```python
from build123d import *

# Parameters (mm, degrees)
F0_W     = 460
F0_H     = 170
F1_DEPTH = 30
F2_W     = 420
F2_H     = 130
F3_DEPTH = 30
F4_W     = 450
F4_H     = 150
F5_DEPTH = 10
F6_W     = 420
F6_H     = 0.1
F7_DEPTH = 0.1


with BuildPart() as f1:
    # F0 (on Top) → F1 (new body)
    with BuildSketch(Plane.XY):
        with Locations((41.152232, -18.289462)):
            Rectangle(F0_W, F0_H)
    extrude(amount=F1_DEPTH)

    # F2 (on face) → F3 (cut, through all)
    with BuildSketch(Plane.XY.offset(30)):
        with Locations((41.152232, -18.289462)):
            Rectangle(F2_W, F2_H)
    extrude(amount=-F3_DEPTH, mode=Mode.SUBTRACT)

    # F4 (on face) → F5 (cut)
    with BuildSketch(Plane(origin=(0, 0, 0), x_dir=(1, 0, 0), z_dir=(0, 0, -1))):
        with Locations((36.152232, 18.289462)):
            Rectangle(F4_W, F4_H)
    extrude(amount=-F5_DEPTH, mode=Mode.SUBTRACT)

    # F6 (on face) → F7 (cut)
    with BuildSketch(Plane(origin=(0, -83.289462, 0), x_dir=(-1, 0, 0), z_dir=(0, 1, 0))):
        with Locations((-41.152232, 20.05)):
            Rectangle(F6_W, F6_H)
    extrude(amount=-F7_DEPTH, mode=Mode.SUBTRACT)


solid = f1.part
```
The model under review builds one solid part; all positions refer to its coordinate system, in mm. A direction names the side the tool comes from. Round coordinates to 2 decimals unless told otherwise and drop trailing zeros. Order: outer loops, then holes, each group sorted by start corner. A loop starts at its lowest first (then second) coordinate and runs counter-clockwise, first axis right, second up. Notation, with made-up numbers: (47, 83.25) -> (78, 83.25) arc R21 ccw to (78, 112.25) -> close; hole circle Ø6 at (9, -31). An arc over 180 degrees is marked (long way). One line per item, written item: value. Start each with the question number.
Q1. Take a section at C-C (x = -43.5). Write out the cut boundary in (y, z), and give its area (4 significant figures).
Q2. Wall thickness on line 1 (Y direction, x = 46.5, z = 22.5); line 2 (X direction, y = -42, z = 26.25); line 3 (Y direction, x = -61, z = 5.5): over which ranges is each line inside the solid? List them lowest first.
Q3. Take a section at B-B (z = 15.25). Write out the cut boundary in (x, y).
Q4. Mouldability with a two-part tool opening along Y and no side actions: class faces 4 (the face through (18, 48, 10)), 5 (the face through (38, -83.289, 15)), 6 (the face through (38, -103.289, 15)), 7 (the face through (-188.848, -19, 18)) as released by +Y, released by -Y, zero draft, split by the parting line, or undercut.
Q5. Take a section at D-D (y = -89). Write out the cut boundary in (x, z).
Q6. Clearance check with flat-ended pins moving along their axes: pin 1 Ø6 at (x, y) = (-0.5, 48.5) entering from -Z; pin 2 Ø5 at (y, z) = (16, 4.5) entering from -X. State where each tip first meets the part, or that it passes through.
Q7. Machinability: for faces 1 (the face through (33, -93.289, 5)), 2 (the face through (38, 46.711, 20)), 3 (the face through (74.15, -93.45, 0)), which of the approach directions +Z, -Z, +X, -X, +Y, -Y give a long, thin tool a straight path to every point of the face, cutting with its end or side? Answer none if there is none.
Q8. Take a section at A-A (y = -31.5). Write out the cut boundary in (x, z), and give its area (3 significant figures).
Reported:
1. outline: (-103.29, 0) -> (-93.29, 0) -> (-93.29, 10) -> (-83.29, 10) -> (-83.29, 20) -> (-83.39, 20) -> (-83.39, 20.1) -> (-83.29, 20.1) -> (-83.29, 30) -> (-103.29, 30) -> close; (46.71, 10) -> (56.71, 10) -> (56.71, 0) -> (66.71, 0) -> (66.71, 30) -> (46.71, 30) -> close
1. area: 1,000 mm2
2. line 1: y = -103.29 to -83.29, 46.71 to 66.71
2. line 2: x = -188.85 to -168.85, 251.15 to 271.15
2. line 3: y = -103.29 to -93.29, 56.71 to 66.71
3. outline: (-188.85, -103.29) -> (271.15, -103.29) -> (271.15, 66.71) -> (-188.85, 66.71) -> close; hole (-168.85, -83.29) -> (251.15, -83.29) -> (251.15, 46.71) -> (-168.85, 46.71) -> close
4. face 4: undercut
4. face 5: undercut
4. face 6: released by -Y
4. face 7: zero draft
5. outline: (-188.85, 10) -> (261.15, 10) -> (261.15, 0) -> (271.15, 0) -> (271.15, 30) -> (-188.85, 30) -> close
6. pin 1: stops at z = 10
6. pin 2: stops at x = 261.15
7. face 1: -Z, -X
7. face 2: +Z, -Z
7. face 3: -Z, +X, -X, +Y, -Y
8. outline: (-188.85, 10) -> (-168.85, 10) -> (-168.85, 30) -> (-188.85, 30) -> close; (251.15, 10) -> (261.15, 10) -> (261.15, 0) -> (271.15, 0) -> (271.15, 30) -> (251.15, 30) -> close
8. area: 900 mm2
